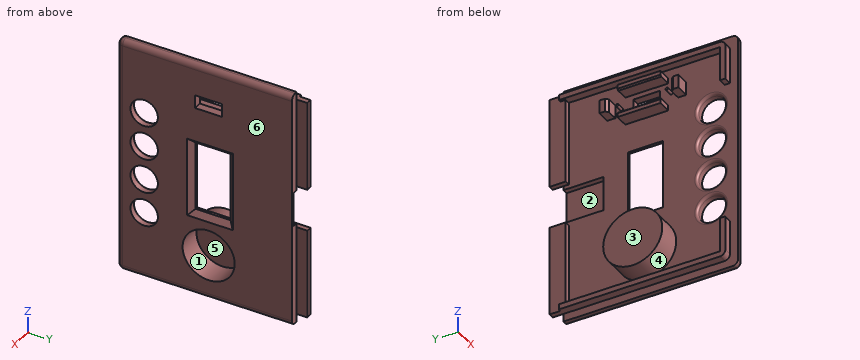
from build123d import *

# Parameters (mm, degrees)
SKETCH014_W     = 65
SKETCH014_H     = 90
SKETCH014_R     = 5.1
SKETCH014_W_2   = 13
SKETCH014_H_2   = 26
PAD010_DEPTH    = 3
SKETCH015_W     = 15
SKETCH015_H     = 13
POCKET004_DEPTH = 2
PAD011_DEPTH    = 3
FILLET009_R     = 2
FILLET010_R     = 2
FILLET011_R     = 2
CHAMFER008_SIZE = 2
CHAMFER009_SIZE = 2
CHAMFER010_SIZE = 2
CHAMFER011_SIZE = 2
FILLET012_R     = 1
FILLET013_R     = 1
FILLET014_R     = 1
FILLET015_R     = 1
FILLET016_R     = 2
FILLET017_R     = 2
SKETCH017_R     = 11
PAD012_DEPTH    = 9
SKETCH019_R     = 9.7
POCKET005_DEPTH = 9
SKETCH020_W     = 10
SKETCH020_H     = 5
POCKET006_DEPTH = 3
SKETCH021_R     = 0.5
PAD013_DEPTH    = 3
SKETCH022_W     = 3
SKETCH022_H     = 5
SKETCH022_W_2   = 16
SKETCH022_H_2   = 2
PAD014_DEPTH    = 5
CHAMFER012_SIZE = 1
CHAMFER013_SIZE = 0.5
CHAMFER014_SIZE = 0.5
CHAMFER015_SIZE = 1
SKETCH023_W     = 6
SKETCH023_H     = 34
PAD015_DEPTH    = 2


with BuildPart() as part:
    # Sketch014 → Pad010 (new body)
    with BuildSketch(Plane.YZ):
        with Locations((32.5, 0)):
            Rectangle(SKETCH014_W, SKETCH014_H)
        with Locations((10, 19.5)):
            Circle(SKETCH014_R, mode=Mode.SUBTRACT)
        with Locations((10, 6.5)):
            Circle(SKETCH014_R, mode=Mode.SUBTRACT)
        with Locations((10, -6.5)):
            Circle(SKETCH014_R, mode=Mode.SUBTRACT)
        with Locations((10, -19.5)):
            Circle(SKETCH014_R, mode=Mode.SUBTRACT)
        with Locations((34.5, 0)):
            Rectangle(SKETCH014_W_2, SKETCH014_H_2, mode=Mode.SUBTRACT)
    extrude(amount=PAD010_DEPTH)

    # Sketch015 (on Face13 of Pad010) → Pocket004 (cut)
    with BuildSketch(Plane(origin=(0, 0, 0), x_dir=(0, 1, 0), z_dir=(-1, 0, 0))):
        with Locations((57.5, 0)):
            Rectangle(SKETCH015_W, SKETCH015_H)
    extrude(amount=-POCKET004_DEPTH, mode=Mode.SUBTRACT)

    # Sketch016 (on Face4 of Pocket004) → Pad011 (join)
    with BuildSketch(Plane(origin=(0, 0, 0), x_dir=(0, 1, 0), z_dir=(-1, 0, 0))):
        Polygon((3, 27), (3, 42), (65, 42), (65, 40), (5, 40), (5, 27), align=None)
        Polygon((3, -27), (3, -42), (65, -42), (65, -40), (5, -40), (5, -27), align=None)
    extrude(amount=PAD011_DEPTH)

    # Fillet009
    fillet009_edges = [part.edges().sort_by_distance(p)[0] for p in [
        (3, 32.5, 45),
    ]]
    fillet(fillet009_edges, radius=FILLET009_R)

    # Fillet010
    fillet010_edges = [part.edges().sort_by_distance(p)[0] for p in [
        (3, 0, -1),
    ]]
    fillet(fillet010_edges, radius=FILLET010_R)

    # Fillet011
    fillet011_edges = [part.edges().sort_by_distance(p)[0] for p in [
        (3, 33.5, -45),
    ]]
    fillet(fillet011_edges, radius=FILLET011_R)

    # Chamfer008
    chamfer008_edges = [part.edges().sort_by_distance(p)[0] for p in [
        (3, 41, 0),
    ]]
    chamfer(chamfer008_edges, length=CHAMFER008_SIZE)

    # Chamfer009
    chamfer009_edges = [part.edges().sort_by_distance(p)[0] for p in [
        (3, 34.5, 13),
    ]]
    chamfer(chamfer009_edges, length=CHAMFER009_SIZE)

    # Chamfer010
    chamfer010_edges = [part.edges().sort_by_distance(p)[0] for p in [
        (3, 35.5, -13),
    ]]
    chamfer(chamfer010_edges, length=CHAMFER010_SIZE)

    # Chamfer011
    chamfer011_edges = [part.edges().sort_by_distance(p)[0] for p in [
        (3, 28, 1),
    ]]
    chamfer(chamfer011_edges, length=CHAMFER011_SIZE)

    # Fillet012
    fillet012_edges = [part.edges().sort_by_distance(p)[0] for p in [
        (0, 4.9, 19.5),
    ]]
    fillet(fillet012_edges, radius=FILLET012_R)

    # Fillet013
    fillet013_edges = [part.edges().sort_by_distance(p)[0] for p in [
        (0, 4.9, 6.5),
    ]]
    fillet(fillet013_edges, radius=FILLET013_R)

    # Fillet014
    fillet014_edges = [part.edges().sort_by_distance(p)[0] for p in [
        (0, 4.9, -6.5),
    ]]
    fillet(fillet014_edges, radius=FILLET014_R)

    # Fillet015
    fillet015_edges = [part.edges().sort_by_distance(p)[0] for p in [
        (0, 4.9, -19.5),
    ]]
    fillet(fillet015_edges, radius=FILLET015_R)

    # Fillet016
    fillet016_edges = [part.edges().sort_by_distance(p)[0] for p in [
        (-1.5, 3, 42),
    ]]
    fillet(fillet016_edges, radius=FILLET016_R)

    # Fillet017
    fillet017_edges = [part.edges().sort_by_distance(p)[0] for p in [
        (-1.5, 3, -42),
    ]]
    fillet(fillet017_edges, radius=FILLET017_R)

    # Sketch017 (on Face1 of Fillet017) → Pad012 (join)
    with BuildSketch(Plane(origin=(0, 0, 0), x_dir=(0, 1, 0), z_dir=(-1, 0, 0))):
        with Locations((34, 28)):
            Circle(SKETCH017_R)
    extrude(amount=PAD012_DEPTH)

    # Sketch019 (on Face33 of Pad012) → Pocket005 (cut)
    with BuildSketch(Plane.YZ.offset(3)):
        with Locations((34, -28)):
            Circle(SKETCH019_R)
    extrude(amount=-POCKET005_DEPTH, mode=Mode.SUBTRACT)

    # Sketch020 (on Face33 of Pocket005) → Pocket006 (cut)
    with BuildSketch(Plane.YZ.offset(3)):
        with Locations((34, 30.5)):
            Rectangle(SKETCH020_W, SKETCH020_H)
    extrude(amount=-POCKET006_DEPTH, mode=Mode.SUBTRACT)

    # Sketch021 (on Face1 of Pocket006) → Pad013 (join)
    with BuildSketch(Plane(origin=(0, 0, 0), x_dir=(0, 1, 0), z_dir=(-1, 0, 0))):
        with Locations((43.25, -30.5)):
            Circle(SKETCH021_R)
        with Locations((24.75, -30.5)):
            Circle(SKETCH021_R)
    extrude(amount=PAD013_DEPTH)

    # Sketch022 (on Face1 of Pad013) → Pad014 (join)
    with BuildSketch(Plane(origin=(0, 0, 0), x_dir=(0, 1, 0), z_dir=(-1, 0, 0))):
        with Locations((47.2, -30.5)):
            Rectangle(SKETCH022_W, SKETCH022_H)
        with Locations((20.8, -30.5)):
            Rectangle(SKETCH022_W, SKETCH022_H)
        with Locations((34, -25.2)):
            Rectangle(SKETCH022_W_2, SKETCH022_H_2)
        with Locations((34, -35.8)):
            Rectangle(SKETCH022_W_2, SKETCH022_H_2)
    extrude(amount=PAD014_DEPTH)

    # Chamfer012
    chamfer012_edges = [part.edges().sort_by_distance(p)[0] for p in [
        (-5, 45.7, 30.5),
    ]]
    chamfer(chamfer012_edges, length=CHAMFER012_SIZE)

    # Chamfer013
    chamfer013_edges = [part.edges().sort_by_distance(p)[0] for p in [
        (-5, 34, 26.2),
    ]]
    chamfer(chamfer013_edges, length=CHAMFER013_SIZE)

    # Chamfer014
    chamfer014_edges = [part.edges().sort_by_distance(p)[0] for p in [
        (-5, 34, 34.8),
    ]]
    chamfer(chamfer014_edges, length=CHAMFER014_SIZE)

    # Chamfer015
    chamfer015_edges = [part.edges().sort_by_distance(p)[0] for p in [
        (-5, 22.3, 30.5),
    ]]
    chamfer(chamfer015_edges, length=CHAMFER015_SIZE)

    # Sketch023 (on Face4 of Chamfer015) → Pad015 (join)
    with BuildSketch(Plane(origin=(0, 0, 0), x_dir=(0, 1, 0), z_dir=(-1, 0, 0))):
        with Locations((66, 25)):
            Rectangle(SKETCH023_W, SKETCH023_H)
        with Locations((66, -25)):
            Rectangle(SKETCH023_W, SKETCH023_H)
    extrude(amount=PAD015_DEPTH)


with BuildPart() as part_1:
    # Body002 placement: moved
    add(part.part.moved(Location((18, 0, 0))))


solid = part_1.part
For this review, take the finished solid that the model builds, in its own axes (mm). Face numbers are marked on the shaded views. A direction names the side the tool comes from. Coordinates: 2 decimals unless noted, no trailing zeros. Loops run counter-clockwise (first coordinate to the right, second up) from the corner with the lowest first, then second, coordinate; pieces in that order, holes last. Notation, with made-up numbers: (7, 71.5) -> (42, 71.5) arc R21 ccw to (42, 96.5) -> close; hole circle Ø1 at (25.25, 78.5). An arc over 180 degrees is marked (long way). Write each question's results on one line, items separated by ' | '.
Q1. Add section C-C, the plane x = 17. Count the separate pieces of the cut face and the enclosed holes in it, then the cut area to 3 significant figures.
Taken from the geometry:
separate pieces: 9 | enclosed holes: 1 | area: 878 mm²
Q2. To check wall thickness, follow line 1 along Z through (x, y) = (17, 65); line 2 along Z through (x, y) = (19.25, 32.5); line 3 along Y through (x, z) = (19, -20). State the ranges of each line that lie inside material, in increasing order. Write a range as [from, to].
Taken from the geometry:
line 1: [-42, -8], [8, 42] | line 2: [-44.98, -37.58], [-18.42, -13.25], [13.25, 28], [33, 44.98] | line 3: [0, 4.92], [15.08, 28.51], [39.49, 65]
Q3. Machinability: for the marked faces 1, 2, 3 and 4, which of the approach directions +Z, -Z, +X, -X, +Y, -Y give a long, thin tool a straight path to every point of the face, cutting with its end or side? Answer none if there is none.
Taken from the geometry:
face 1: +X | face 2: -X, +Y | face 3: +Z, -Z, -X, +Y, -Y | face 4: -X
Q4. Add section D-D, the plane z = 39. State the section outline as (x, y) points.
Taken from the geometry:
outline: (15, 3) -> (18, 3) -> (18, 0) -> (19, 0) arc R2 ccw to (21, 2) -> (21, 65) -> (18, 65) -> (18, 69) -> (16, 69) -> (16, 63) -> (18, 63) -> (18, 5) -> (15, 5) -> close
Q5. For pin 1 Ø1.1 at (y, z) = (25, 30.5) entering from -X; pin 2 Ø6 at (y, z) = (30.5, -31) entering from +X; pin 3 Ø1.2 at (y, z) = (67.5, -22) entering from +X; pin 4 Ø2 at (x, y) = (19.5, 61) entering from +Z, all flat-tipped, find the tip position at first contact; note any pin that passes through.
Taken from the geometry:
pin 1: x = 15 | pin 2: x = 12 | pin 3: x = 18 | pin 4: z = 45
Q6. Add section A-A, the plane z = 19.5. State the section outline as (x, y) points.
Taken from the geometry:
outline: (16, 63) -> (18, 63) -> (18, 16.1) arc R1 ccw to (19, 15.1) -> (21, 15.1) -> (21, 65) -> (18, 65) -> (18, 69) -> (16, 69) -> close; (18, 0) -> (19, 0) arc R2 ccw to (21, 2) -> (21, 4.9) -> (19, 4.9) arc R1 ccw to (18, 3.9) -> close
Q7. Mouldability with a two-part tool opening along Z and no side actions: class the marked faces 5 and 6 as +Z half, -Z half, draft (parallel to the pull), parting line (faces both ways), or undercut.
Taken from the geometry:
face 5: undercut | face 6: draft
Q8. Add section B-B, the plane y = 17.5. State the section outline as (x, z) points.
Taken from the geometry:
outline: (15, -42) -> (18, -42) -> (18, -45) -> (19, -45) arc R2 ccw to (21, -43) -> (21, 43) arc R2 ccw to (19, 45) -> (18, 45) -> (18, 42) -> (15, 42) -> (15, 40) -> (18, 40) -> (18, -40) -> (15, -40) -> close
